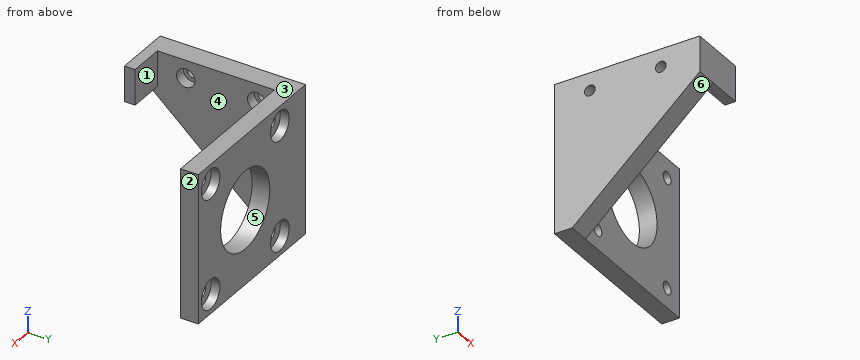
Autodesk Inventor part; units mm, degrees
ref_plane "YZ Plane" through (0, 0, 0) normal (1, 0, 0) x (0, 1, 0)
ref_plane "XZ Plane" through (0, 0, 0) normal (0, 1, 0) x (-1, 0, 0)
ref_plane "XY Plane" through (0, 0, 0) normal (0, 0, 1) x (1, 0, 0)
sketch "Sketch1" plane through (0, 0, 0) normal (0, 1, 0) x (-1, 0, 0)
  line L0 (-21, -21) -> (21, -21)
  line L1 (21, -21) -> (21, 21)
  line L2 (21, 21) -> (-21, 21)
  line L3 (-21, 21) -> (-21, -21)
  line L4 (-21, -21) -> (21, 21) construction
  line L5 (21, -21) -> (-21, 21) construction
  circle A0 centre (15.5, 15.5) radius 1.75
  circle A1 centre (15.5, -15.5) radius 1.75
  circle A2 centre (-15.5, -15.5) radius 1.75
  circle A3 centre (-15.5, 15.5) radius 1.75
  circle A4 centre (0, 0) radius 11
  circle A5 centre (0, 0) radius 4 construction
  line L6 (21, -17) -> (17, -21)
  line L7 (21, 17) -> (17, 21)
  line L8 (-17, -21) -> (-21, -17)
  line L9 (-21, 17) -> (-17, 21)
  circle A6 centre (0, 0) radius 2.5 construction
  circle A7 centre (44, -10) radius 4 construction
  line L10 (44, -10) -> (44, 10) construction
  circle A8 centre (44, -10) radius 7.5 construction
  circle A9 centre (44, 10) radius 11.15 construction
  circle A10 centre (44, 10) radius 3.5 construction
  circle A11 centre (52, 10) radius 1.5 construction
  line L11 (52, 10) -> (44, 10) construction
  circle A12 centre (44, 18) radius 1.5 construction
  circle A13 centre (36, 10) radius 1.5 construction
  circle A14 centre (44, 2) radius 1.5 construction
  circle A15 centre (44, 10) radius 5.1 construction
  line L12 (44, 0) -> (21, 0) construction
  circle A16 centre (-15.5, -15.5) radius 4.15
  circle A17 centre (-15.5, 15.5) radius 4.15
  circle A18 centre (15.5, -15.5) radius 4.15
  circle A19 centre (15.5, 15.5) radius 4.15
  line L13 (21, -21) -> (24, -21)
  line L14 (21, 21) -> (21, -21)
  line L15 (27, -21) -> (27, 21)
  line L16 (24, -21) -> (27, -21)
  line L17 (21, 21) -> (27, 21)
  dimension "d0" = 42
  dimension "d1" = 31
  dimension "d2" = 31
  dimension "d3" = 31
  dimension "d4" = 31
  dimension "d5" = 3.5
  dimension "d6" = 3.5
  dimension "d7" = 3.5
  dimension "d8" = 3.5
  dimension "d9" = 22
  dimension "d10" = 8
  dimension "d11" = 4
  dimension "d12" = 4
  dimension "d13" = 4
  dimension "d14" = 4
  dimension "d15" = 4
  dimension "d16" = 4
  dimension "d17" = 4
  dimension "d18" = 5
  dimension "d21" = 8
  dimension "d23" = 20
  dimension "d24" = 15
  dimension "d28" = 22.3
  dimension "d29" = 7
  dimension "d30" = 3
  dimension "d31" = 8
  dimension "d32" = 360
  dimension "d33" = 10.2
  dimension "d36" = 2.4
  dimension "d38" = 2.4
  dimension "d39" = 2.4
  dimension "d40" = 2.4
  dimension "d46" = 17
  dimension "d47" = 6
extrude "Extrusion1" add sketch "Sketch1" along normal blind 5 contours L3 L8 L0 | L8 L3 L9 L2 L7 L1 L6 L0 | L6 L1 L0 | L3 L2 L9 | L1 L17 L15 L16 L13 | L7 L2 L1
extrude "Extrusion2" add sketch "Sketch1" along normal blind 2.5 contours A16 | A17 | A18 | A19
ref_plane "Work Plane1" through (-21, -30, 21) normal (1, 0, 0) x (0, 0, -1)
sketch "Sketch2" plane through (-21, -30, 21) normal (1, 0, 0) x (0, 0, -1)
  line L0 (42, 30) -> (42, -6)
  line L1 (20, 30) -> (20, -6) construction
  circle A0 centre (5, 25) radius 2.6
  circle A1 centre (5, 25) radius 1.5
  circle A2 centre (5, 5) radius 2.6
  circle A3 centre (5, 5) radius 1.5
  line L2 (0, 30) -> (0, 35)
  line L3 (0, 30) -> (42, 30)
  line L4 (0, 30) -> (42, 30)
  line L5 (42, 30) -> (42, -6)
  line L6 (42, -6) -> (0, -6)
  line L7 (0, -6) -> (0, 30)
  line L8 (42, 30) -> (42, 35)
  line L9 (42, 30) -> (20, -6) construction
  line L10 (20, 0) -> (0, 0) construction
  line L11 (0, -6) -> (10, -6)
  line L12 (10, -6) -> (10, -3)
  line L13 (10, -3) -> (0, -3)
  line L14 (0, -3) -> (0, -6)
  line L15 (18, 3) -> (24, 3) construction
  line L16 (24, 3) -> (24, -3) construction
  line L17 (24, -3) -> (18, -3) construction
  line L18 (18, -3) -> (18, 3) construction
  line L19 (42, 30) -> (10, -6)
  point P0 (21, 30)
  point P1 (0, -4.5)
  point P2 (0, -3)
  point P3 (10, -6)
  point P4 (10, -6)
  dimension "d51" = 5.2
  dimension "d52" = 3
  dimension "d59" = 5.2
  dimension "d60" = 3
  dimension "d64" = 5
  dimension "d66" = 5
  dimension "d67" = 20
  dimension "d68" = 25
  dimension "d69" = 20
  dimension "d70" = 36
  dimension "d71" = 30
  dimension "d72" = 10
  dimension "d73" = 3
  dimension "d76" = 18
  dimension "d77" = 6
  dimension "d78" = 6
  dimension "d79" = 3
extrude "Extrusion4" add sketch "Sketch2" against normal up to surface (6 mm away) contours L19 L12 L13 L7 L3 | L6 L7 L13 L12
extrude "Extrusion5" add sketch "Sketch2" along normal blind 3 from surface at -6 contours A0 | A2
extrude "Extrusion6" add sketch "Sketch2" along normal blind 10 contours L6 L7 L13 L12
equation "\"d2\" = d1"
equation "\"d3\" = d1"
equation "\"d4\" = d1"
equation "\"d6\" = d5"
equation "\"d7\" = d5"
equation "\"d8\" = d5"
equation "\"d12\" = d11"
equation "\"d13\" = d11"
equation "\"d14\" = d11"
equation "\"d15\" = d11"
equation "\"d16\" = d11"
equation "\"d17\" = d11"
properties part number "CoreXY Stepper Holder"
Source: CAD feature listing. Evaluate the final solid. Frame: model axes, mm. Face numbers are marked on the shaded views. A direction names the side the tool comes from. Give positions to 0.01 mm unless a question says otherwise; leave off trailing zeros. Write each loop counter-clockwise with the first axis right and the second up, starting at its lowest first coordinate (ties: lowest second). Pieces come first, ordered by that corner, then holes. Notation, with made-up numbers: M 35,13 L 43,13 A14 ccw 43,26 Z; hole C -17,50.25 d10. An arc over 180 degrees is marked long. Return JSON: item names as keys, results as strings. Group by question number.
1) Pull-direction query (Z, two-part tool) for the marked faces 3, 4, 5 and 6; classes: pulls with the +Z half, pulls with the -Z half, needs draft (parallel to the pull), parting line crosses it, or undercut.
2) Cut plane C-C, the plane z = -14.5. Output: boundary loops of the cut face in (x, y), plus the area to 3 significant figures.
3) Material intervals for line 1 along Z through (x, y) = (15.5, 4.55); line 2 along Y through (x, z) = (-25, 16); line 3 along Y through (x, z) = (-22, 16), sorted ascending. Write a range as [from, to].
4) Set-up query: the marked faces 1 and 2. Return all of +Z, -Z, +X, -X, +Y, -Y with unobstructed straight access to the full face (end or side cutting, diameter ignored); none if empty.
5) Pin query (flat end, axial travel): P1, Ø3.5, axis at y = -34, z = 15, coming from the +X side; P2, Ø10, axis at x = 7, y = -7.5, coming from the -Z side; P3, Ø2.5, axis at x = -14, y = -34.5, coming from the -Z side; P4, Ø2, axis at x = -9, z = -10.5, coming from the -Y side. Return the tip coordinate at first contact, or that it passes through.
6) Cut plane D-D, the plane y = -9. Output: boundary loops of the cut face in (x, z).
7) Cut plane B-B, the plane z = 6.5. Output: boundary loops of the cut face in (x, y).
8) Cut plane A-A, the plane x = -15.5. Output: boundary loops of the cut face in (y, z).
Recorded:
{
 "1": {"face 3": "pulls with the +Z half", "face 4": "needs draft", "face 5": "undercut", "face 6": "pulls with the -Z half"},
 "2": {"outline": "M -27,-7.31 L -21,-7.31 L -21,0 L -16.94,0 L -16.94,2.5 L -19.53,2.5 L -19.53,5 L -27,5 Z; M -14.06,0 L 14.06,0 L 14.06,2.5 L 11.47,2.5 L 11.47,5 L -11.47,5 L -11.47,2.5 L -14.06,2.5 Z; M 16.94,0 L 21,0 L 21,5 L 19.53,5 L 19.53,2.5 L 16.94,2.5 Z", "area": "229 mm²"},
 "3": {"line 1": "z = [-21, -19.65], [-11.35, 11.35], [19.65, 21]", "line 2": "y = [-36, -26.5], [-23.5, -6.5], [-3.5, 5]", "line 3": "y = [-36, -27.6], [-22.4, -7.6], [-2.4, 5]"},
 "4": {"face 1": "+Z, -Z, +X", "face 2": "+Z, -Z, +X, +Y, -Y"},
 "5": {"P1": "stops at x = -11", "P2": "passes through", "P3": "stops at z = 11", "P4": "stops at y = 0"},
 "6": {"outline": "M -27,-13 L -21,-13 L -21,21 L -27,21 Z"},
 "7": {"outline": "M -27,-30.94 L -21,-30.94 L -21,0 L -8.87,0 L -8.87,5 L -27,5 Z; M 8.87,0 L 21,0 L 21,5 L 8.87,5 Z"},
 "8": {"outline": "M -36,11 L -33,11 L -33,21 L -36,21 Z; M 0,-21 L 5,-21 L 5,-19.65 L 2.5,-19.65 L 2.5,-17.25 L 0,-17.25 Z; M 0,-13.75 L 2.5,-13.75 L 2.5,-11.35 L 5,-11.35 L 5,11.35 L 2.5,11.35 L 2.5,13.75 L 0,13.75 Z; M 0,17.25 L 2.5,17.25 L 2.5,19.65 L 5,19.65 L 5,21 L 0,21 Z"}
}
